Autodesk Inventor part; units mm, degrees
ref_plane "YZ Plane" through (0, 0, 0) normal (1, 0, 0) x (0, 1, 0)
ref_plane "XZ Plane" through (0, 0, 0) normal (0, 1, 0) x (-1, 0, 0)
ref_plane "XY Plane" through (0, 0, 0) normal (0, 0, 1) x (1, 0, 0)
sketch "Sketch1" plane through (0, 0, 0) normal (0, 0, 1) x (1, 0, 0)
  line L0 (-15.25, 6.5) -> (-15.25, -6.5) construction
  line L1 (18.75, 6.5) -> (-15.25, 6.5) construction
  line L2 (18.75, -6.5) -> (18.75, 6.5) construction
  line L3 (-15.25, -6.5) -> (18.75, -6.5) construction
  line L4 (9.8054, 8.5) -> (19.75, 8.5) construction
  arc A0 (9.8054, 8.5) -> (9.8054, -8.5) centre (-3.75, 0) ccw construction
  line L5 (19.75, -8.5) -> (9.8054, -8.5) construction
  line L6 (19.75, 8.5) -> (19.75, -8.5) construction
  circle A1 centre (-3.75, 0) radius 16
  point P0 (0, 0)
extrude "Extrusion1" add sketch "Sketch1" along normal blind 7
sketch "Sketch4" plane through (-3.75, 0, 7) normal (0, 0, 1) x (1, 0, 0)
  line L0 (0, 0) -> (-50, 0) construction
  line L1 (0, 10) -> (-50, 10)
  line L2 (-50, -10) -> (0, -10)
  arc A0 (0, -10) -> (0, 10) centre (0, 0) ccw
  arc A1 (-50, 10) -> (-50, -10) centre (-50, 0) ccw
  point P0 (3.75, 0)
  point P1 (-25, 0)
  dimension "d6" = 50
  dimension "d7" = 10
extrude "Extrusion3" add sketch "Sketch4" against normal blind 3
sketch "Sketch5" plane through (0, 0, 7) normal (0, 0, 1) x (1, 0, 0)
  arc A0 (-53.75, 10) -> (-53.75, -10) centre (-53.75, 0) ccw construction
  line L0 (-53.75, -10) -> (-16.24, -10) construction
  line L1 (-16.24, 10) -> (-53.75, 10) construction
  line L2 (-45.75, -22.5) -> (-61.75, -22.5)
  line L3 (-61.75, -22.5) -> (-61.75, 22.5)
  line L4 (-61.75, 22.5) -> (-45.75, 22.5)
  line L5 (-45.75, 22.5) -> (-45.75, -22.5)
  line L6 (-61.75, -22.5) -> (-45.75, 22.5) construction
  line L7 (-45.75, -22.5) -> (-61.75, 22.5) construction
  line L8 (-77.75, -22.5) -> (-61.75, -22.5)
  line L9 (-61.75, -22.5) -> (-61.75, 22.5)
  line L10 (-61.75, 22.5) -> (-77.75, 22.5)
  line L11 (-77.75, 22.5) -> (-77.75, -22.5)
  point P0 (0, 0)
  dimension "d10" = 45
  dimension "d11" = 16
  dimension "d12" = 16
extrude "Extrusion4" cut sketch "Sketch5" against normal blind 3 contours L8 L11 L10 L3
extrude "Extrusion5" add sketch "Sketch5" against normal blind 3 contours L2 L3 L4 L5
sketch "Sketch6" plane through (0, 0, 7) normal (0, 0, 1) x (1, 0, 0)
  line L0 (-53.75, -22.5) -> (-61.75, -22.5)
  line L1 (-61.75, -22.5) -> (-61.75, 22.5)
  line L2 (-61.75, 22.5) -> (-53.75, 22.5)
  line L3 (-53.75, 22.5) -> (-53.75, -22.5)
  line L4 (-61.75, -22.5) -> (-61.75, 22.5) construction
  line L5 (-45.75, -22.5) -> (-61.75, -22.5)
  line L6 (-61.75, 22.5) -> (-45.75, 22.5)
  point P0 (0, 0)
  dimension "d17" = 8
extrude "Extrusion6" add sketch "Sketch6" along normal blind 13
sketch "Sketch7" plane through (0, 0, 7) normal (0, 0, 1) x (1, 0, 0)
  line L0 (-43.25, -5.5) -> (-51.25, -5.5)
  line L1 (-51.25, -5.5) -> (-51.25, 5.5)
  line L2 (-51.25, 5.5) -> (-43.25, 5.5)
  line L3 (-43.25, 5.5) -> (-43.25, -5.5)
  line L4 (-53.75, -22.5) -> (-53.75, 22.5)
  line L5 (-53.75, -22.5) -> (-51.25, -5.5) construction
  line L6 (-51.25, 5.5) -> (-53.75, 22.5) construction
  point P0 (0, 0)
  dimension "d20" = 2.5
  dimension "d21" = 8
  dimension "d22" = 11
extrude "Extrusion7" cut sketch "Sketch7" against normal through all
sketch "Sketch8" plane through (0, 0, 20) normal (0, 0, 1) x (1, 0, 0)
  line L0 (-59.75, -22.5) -> (-61.75, -22.5)
  line L1 (-61.75, -22.5) -> (-61.75, 22.5)
  line L2 (-61.75, 22.5) -> (-59.75, 22.5)
  line L3 (-59.75, 22.5) -> (-59.75, -22.5)
  line L4 (-61.75, 22.5) -> (-61.75, -22.5)
  line L5 (-61.75, -22.5) -> (-53.75, -22.5)
  line L6 (-53.75, 22.5) -> (-61.75, 22.5)
  point P0 (0, 0)
  dimension "d25" = 2
extrude "Extrusion8" cut sketch "Sketch8" against normal through all
ref_plane "Work Plane1" through (-3.75, 0, 3.5) normal (0, 0, -1) x (-1, 0, 0)
sketch "Sketch12" plane through (0, 0, 7) normal (0, 0, 1) x (1, 0, 0)
  arc A0 (-16.24, -10) -> (-16.24, 10) centre (-3.75, 0) ccw
  circle A1 centre (-3.75, 0) radius 3
  point P0 (0, 0)
  dimension "d46" = 6
extrude "Extrusion11" cut sketch "Sketch12" against normal through all
sketch "Sketch13" plane through (-53.75, -22.5, 7) normal (1, 0, 0) x (0, 0, -1)
  line L0 (0, 45) -> (-13, 45)
  line L1 (0, 0) -> (-13, 0)
  line L2 (-13, 0) -> (-13, 45) construction
  line L3 (0, 12.5) -> (0, 0) construction
  line L4 (0, 45) -> (0, 32.5) construction
  line L5 (-6.5, 3.5) -> (-13, 3.5) construction
  line L6 (-6.5, 3.5) -> (0, 3.5) construction
  line L7 (-6.5, 41.5) -> (-13, 41.5) construction
  line L8 (-6.5, 41.5) -> (0, 41.5) construction
  point P0 (7, 22.5)
  dimension "d37" = 3.5
  dimension "d38" = 3.5
hole "Hole1" at (-53.75, -19, 13.5) at (-53.75, 19, 13.5) direction (-1, 0, 0) diameter 2 depth 5 tip angle 118
sketch "Sketch14" plane through (-3.75, 0, 0) normal (0, 0, -1) x (-1, 0, 0)
  circle A0 centre (0, 0) radius 7
  point P0 (-3.75, 0)
  dimension "d47" = 14
extrude "Extrusion12" cut sketch "Sketch14" against normal blind 5
equation "\"d38\" = d37"
properties part number "arm" material "Ogólne"
Geometry check sheet. Reference: the model listing, model coordinates, mm. A direction names the side the tool comes from. Coordinates: 2 decimals unless noted, no trailing zeros. Order: outer loops, then holes, each group sorted by start corner. A loop starts at its lowest first (then second) coordinate and runs counter-clockwise, first axis right, second up. Notation, with made-up numbers: M 52,-5 L 90,-5 A25 ccw 90,22 Z; hole C -5,66.5 d3. An arc over 180 degrees is marked long. Answer as a JSON object with one key per item and string values.
Q1. Cross-section at D-D on x = -21. Record the cut outline in (y, z), and give its area (3 significant figures).
Results are:
{"outline": "M -10,4 L 10,4 L 10,7 L -10,7 Z", "area": "60.0 mm²"}
Q2. Cross-section at C-C on x = -3.75. Record the cut outline in (y, z).
Results are:
{"outline": "M -16,0 L -7,0 L -7,5 L -3,5 L -3,7 L -16,7 Z; M 3,5 L 7,5 L 7,0 L 16,0 L 16,7 L 3,7 Z"}
Q3. Release check for a two-part mould opening along X. For faces 1 (the flat face through (3, -3, 0)), 2 (the flat face through (-53.75, 0, 13)), 3 (the flat face through (-47, -5.5, 6)), 4 (the flat face through (-45.75, -16, 6)) record: released by +X, released by -X, zero draft, split by the parting line, or undercut.
Results are:
{"face 1": "zero draft", "face 2": "released by +X", "face 3": "undercut", "face 4": "undercut"}
Q4. Tool access check on faces 5 (the flat face through (-21, 0, 7)), 6 (the cylindrical face through (-56.28, -18.11, 13.04)), 7 (the flat face through (-51.25, 0, 6)), 8 (the cylindrical face through (11.51, -4.81, 3.45)). Record the directions out of +Z, -Z, +X, -X, +Y, -Y that give a thin tool (end or side, any length) a straight path to the whole face; none if there is none.
Results are:
{"face 5": "+Z, +X, +Y, -Y", "face 6": "+X", "face 7": "+Z, -Z", "face 8": "-Z"}
Q5. Depth check by flat-ended pin: pin 1 Ø1.5 at (y, z) = (-13, 5.5) entering from +X; pin 2 Ø2.5 at (y, z) = (19, 13.5) entering from +X; pin 3 Ø10 at (x, z) = (-35.5, 7) entering from -Y. Enter the tip coordinate at first touch or a pass-through.
Results are:
{"pin 1": "stops at x = 6.54", "pin 2": "stops at x = -53.75", "pin 3": "stops at y = -10"}
Q6. Cross-section at A-A on x = -48. Record the cut outline in (y, z), and give its area (3 significant figures).
Results are:
{"outline": "M -22.5,4 L -5.5,4 L -5.5,7 L -22.5,7 Z; M 5.5,4 L 22.5,4 L 22.5,7 L 5.5,7 Z", "area": "102 mm²"}
Q7. Scan lines: line 1 (Y direction, x = -54.8, z = 13.5); line 2 (Y direction, x = -3.75, z = 5.85); line 3 (Y direction, x = -3.75, z = 3.75). Record each from-to range of solid material in increasing order.
Results are:
{"line 1": "y = -22.5 to -20, -18 to 18, 20 to 22.5", "line 2": "y = -16 to -3, 3 to 16", "line 3": "y = -16 to -7, 7 to 16"}
Q8. Cross-section at B-B on y = 0. Record the cut outline in (x, z), and give its area (3 significant figures).
Results are:
{"outline": "M -59.75,4 L -51.25,4 L -51.25,7 L -53.75,7 L -53.75,20 L -59.75,20 Z; M -43.25,4 L -19.75,4 L -19.75,0 L -10.75,0 L -10.75,5 L -6.75,5 L -6.75,7 L -43.25,7 Z; M -0.75,5 L 3.25,5 L 3.25,0 L 12.25,0 L 12.25,7 L -0.75,7 Z", "area": "316 mm²"}
